from build123d import *

# Parameters (mm, degrees)
CROQUIS2_R              = 17.25
SALIENTE_EXTRUIR1_DEPTH = 794.82
CROQUIS4_R              = 29.5
SALIENTE_EXTRUIR2_DEPTH = 33.5
REDONDEO2_R             = 22


with BuildPart() as part:
    # Croquis2 → Saliente-Extruir1 (new body)
    with BuildSketch(Plane(origin=(0, 0, 0), x_dir=(1, 0, 0), z_dir=(0, 1, 0))):
        with Locations(Location((0, 0, 0), (0, 0, 270))):
            Circle(CROQUIS2_R)
    extrude(amount=SALIENTE_EXTRUIR1_DEPTH)

    # Croquis4 → Saliente-Extruir2 (add)
    with BuildSketch(Plane.XZ):
        with Locations(Location((0, 0, 0), (0, 0, 270))):
            Circle(CROQUIS4_R)
    extrude(amount=SALIENTE_EXTRUIR2_DEPTH)

    # Redondeo2
    redondeo2_edges = [part.edges().sort_by_distance(p)[0] for p in [
        (0, -33.5, 29.5),
    ]]
    fillet(redondeo2_edges, radius=REDONDEO2_R)


solid = part.part
The listing builds one solid part. Answer for the finished solid, in the listing's coordinates (mm). A direction names the side the tool comes from. Round coordinates to 2 decimals unless told otherwise and drop trailing zeros. Order: outer loops, then holes, each group sorted by start corner. A loop starts at its lowest first (then second) coordinate and runs counter-clockwise, first axis right, second up. Notation, with made-up numbers: (-38, 82.25) - (6, 82.25) arc R31 ccw to (6, 113.25) - close; hole circle Ø7 at (-10.75, 30.5). An arc over 180 degrees is marked (long way). Write item = value, one per line. Start each with the question number.
1) For faces 1 (the flat face through (-13, 0, -13)), 2 (the flat face through (0, 794.82, 0)), determine the directions among +Z, -Z, +X, -X, +Y, -Y from which every point of the face is accessible in a straight line to the end or side of a thin tool.
2) Section A-A, the plane y = 629.5 is taken. Write down the section's boundary in (x, z), plus the area to 3 significant figures.
3) Straight lines are drawn through the part: L1, parallel to Y at x = -1, z = 10; L2, parallel to X at y = 315.5, z = 15.5; L3, parallel to Y at x = 15, z = -18. For each, find the intervals that lie inside material, in ascending order.
4) Given pin 1 (1.5 mm diameter, centred on x = 22, z = -12.5, fed in from +Y); pin 2 (3 mm diameter, centred on x = -22.5, z = -15.5, fed in from -Y); pin 3 (12 mm diameter, centred on x = 21, y = 122.5, fed in from +Z); pin 4 (4 mm diameter, centred on x = 12.5, z = -13, fed in from +Y), each flat-ended and moving along its own axis, determine where each tip first touches the part or whether it passes through.
Results list:
q1.face_1 = +Y
q1.face_2 = +Z, -Z, +X, -X, +Y
q2.outline = circle Ø34.5 at (0, 0)
q2.area = 935 mm^2
q3.L1 = -33.35 to 794.82
q3.L2 = -7.57 to 7.57
q3.L3 = -26.67 to 0
q4.pin_1 = 0
q4.pin_2 = -23.68
q4.pin_3 = 8.52
q4.pin_4 = 794.82
